Read the model definition and answer for the solid it produces. Units are mm, in the model's axes. Face numbers are marked on the shaded views. Round coordinates to 2 decimals unless told otherwise and drop trailing zeros. Loops run counter-clockwise (first coordinate to the right, second up) from the corner with the lowest first, then second, coordinate; pieces in that order, holes last. Notation, with made-up numbers: (39.5, -8.75) - (54.5, -8.75) arc R11 ccw to (54.5, 10.25) - close; hole circle Ø8 at (-28, 6). An arc over 180 degrees is marked (long way). Answer as CSV lines item,"result".
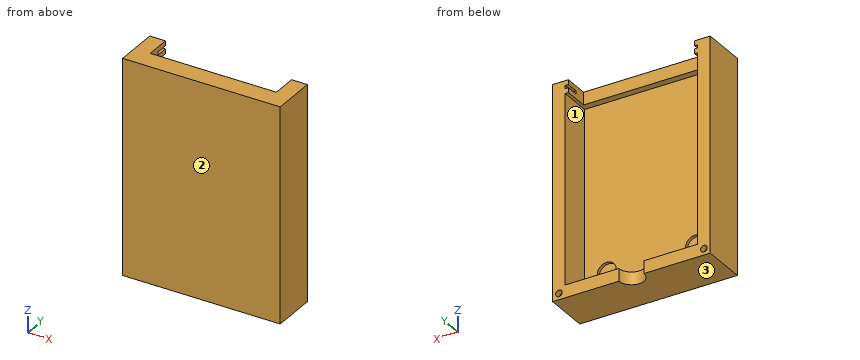
```python
from build123d import *

# Parameters (mm, degrees)
IZIM1_W                     = 25
IZIM1_H                     = 34
Y_KSEKLIK_EKSTR_ZYON1_DEPTH = 7.04
IZIM2_W                     = 21
IZIM2_H                     = 30
KES_EKSTR_ZYON1_DEPTH       = 5.04
IZIM3_W                     = 20
IZIM3_H                     = 3.94
KES_EKSTR_ZYON2_DEPTH       = 36.068669778
FEDER1_START                = -1.1
FEDER1_OUTLINE_W            = 1.1
FEDER1_OUTLINE_H            = 1.1
FEDER1_DEPTH                = 2.2
IZIM7_W                     = 1
IZIM7_H                     = 0.5
KES_EKSTR_ZYON3_DEPTH       = 2
IZIM9_R                     = 2
KES_EKSTR_ZYON4_DEPTH       = 2
IZIM10_R                    = 1.5
KES_EKSTR_ZYON5_DEPTH       = 0.5
IZIM11_R                    = 0.525
KES_EKSTR_ZYON6_DEPTH       = 1.01


# Read off the part's stored shape, not the designer's step: Feder1
with BuildPart() as part:
    # Çizim1 → Yükseklik-Ekstrüzyon1 (new body)
    with BuildSketch(Plane(origin=(0, 7.04, 0), x_dir=(1, 0, 0), z_dir=(0, 1, 0))):
        Rectangle(IZIM1_W, IZIM1_H)
    extrude(amount=-Y_KSEKLIK_EKSTR_ZYON1_DEPTH)

    # Çizim2 → Kes-Ekstrüzyon1 (cut)
    with BuildSketch(Plane(origin=(0, 7.04, 0), x_dir=(-1, 0, 0), z_dir=(0, 1, 0))):
        Rectangle(IZIM2_W, IZIM2_H)
    extrude(amount=-KES_EKSTR_ZYON1_DEPTH, mode=Mode.SUBTRACT)

    # Çizim3 → Kes-Ekstrüzyon2 (cut, through all)
    with BuildSketch(Plane(origin=(0, 0, 15), x_dir=(-1, 0, 0), z_dir=(0, 0, -1))):
        with Locations((0, 5.07)):
            Rectangle(IZIM3_W, IZIM3_H)
    extrude(amount=-KES_EKSTR_ZYON2_DEPTH, mode=Mode.SUBTRACT)

    # Feder1 outline → Feder1 (add)
    with BuildSketch(Plane(origin=(0, 0, 0), x_dir=(0, 0, -1), z_dir=(1, 0, 0)).offset(FEDER1_START)):
        with Locations((14.45, 2.55)):
            Rectangle(FEDER1_OUTLINE_W, FEDER1_OUTLINE_H)
    extrude(amount=FEDER1_DEPTH)

    # Çizim7 → Kes-Ekstrüzyon3 (cut)
    with BuildSketch(Plane(origin=(0, 7.04, 0), x_dir=(1, 0, 0), z_dir=(0, 1, 0))):
        with Locations((-10, -16)):
            Rectangle(IZIM7_W, IZIM7_H)
        with Locations((10, -16)):
            Rectangle(IZIM7_W, IZIM7_H)
    extrude(amount=-KES_EKSTR_ZYON3_DEPTH, mode=Mode.SUBTRACT)

    # Çizim9 → Kes-Ekstrüzyon4 (cut)
    with BuildSketch(Plane(origin=(0, 0, -17), x_dir=(-1, 0, 0), z_dir=(0, 0, -1))):
        with Locations((0, 7.04)):
            Circle(IZIM9_R)
    extrude(amount=-KES_EKSTR_ZYON4_DEPTH, mode=Mode.SUBTRACT)

    # Çizim10 → Kes-Ekstrüzyon5 (cut)
    with BuildSketch(Plane(origin=(0, 2, 0), x_dir=(1, 0, 0), z_dir=(0, 1, 0))):
        with Locations(Location((-7, 11.5, 0), (0, 0, 270))):
            Circle(IZIM10_R)
        with Locations(Location((7, 11.5, 0), (0, 0, 270))):
            Circle(IZIM10_R)
    extrude(amount=-KES_EKSTR_ZYON5_DEPTH, mode=Mode.SUBTRACT)

    # Çizim11 → Kes-Ekstrüzyon6 (cut)
    with BuildSketch(Plane(origin=(0, 7.04, 0), x_dir=(1, 0, 0), z_dir=(0, 1, 0))):
        with Locations(Location((-11.5, 16, 0), (0, 0, 270))):
            Circle(IZIM11_R)
        with Locations(Location((11.5, 16, 0), (0, 0, 270))):
            Circle(IZIM11_R)
    extrude(amount=-KES_EKSTR_ZYON6_DEPTH, mode=Mode.SUBTRACT)


solid = part.part
```
1) A cutting plane is placed at A-A, the plane z = -16. Determine the outline of the cut face in (x, y) (3 decimals).
Entries:
outline,"(-12.5, 0) - (12.5, 0) - (12.5, 7.04) - (12.025, 7.04) - (12.025, 6.03) - (10.975, 6.03) - (10.975, 7.04) - (2, 7.04) arc R2 cw to (-2, 7.04) - (-10.975, 7.04) - (-10.975, 6.03) - (-12.025, 6.03) - (-12.025, 7.04) - (-12.5, 7.04) - close"
2) A cutting plane is placed at D-D, the plane x = -9. Determine the outline of the cut face in (y, z), plus the area to 3 significant figures.
Entries:
outline,"(0, -17) - (7.04, -17) - (7.04, -15) - (2, -15) - (2, 15) - (3.1, 15) - (3.1, 17) - (0, 17) - close"
area,"80.3 mm^2"
3) A cutting plane is placed at B-B, the plane x = 7. Determine the outline of the cut face in (y, z), plus the area to 3 significant figures.
Entries:
outline,"(0, -17) - (7.04, -17) - (7.04, -15) - (2, -15) - (2, -13) - (1.5, -13) - (1.5, -10) - (2, -10) - (2, 15) - (3.1, 15) - (3.1, 17) - (0, 17) - close"
area,"78.8 mm^2"
4) A cutting plane is placed at C-C, the plane z = -11.5. Determine the outline of the cut face in (x, y).
Entries:
outline,"(-12.5, 0) - (12.5, 0) - (12.5, 7.04) - (10.5, 7.04) - (10.5, 2) - (8.5, 2) - (8.5, 1.5) - (5.5, 1.5) - (5.5, 2) - (-5.5, 2) - (-5.5, 1.5) - (-8.5, 1.5) - (-8.5, 2) - (-10.5, 2) - (-10.5, 7.04) - (-12.5, 7.04) - close"
5) Find the intervals of material crossed by line 1 (X direction, y = 1.95, z = -11.5); line 2 (X direction, y = 3.75, z = 8); line 3 (Z direction, x = 1, y = 3), in increasing order.
Entries:
line 1,"x = -12.5 to -8.5, -5.5 to 5.5, 8.5 to 12.5"
line 2,"x = -12.5 to -10.5, 10.5 to 12.5"
line 3,"z = -17 to -13.9, 15 to 17"
6) Each of these flat-tipped pins is pushed along its axis until it touches: P1, Ø0.9, axis at x = -11.5, z = -16, coming from the +Y side; P2, Ø0.6, axis at x = 0, z = -14.5, coming from the +Y side; P3, Ø1.5, axis at x = 3, y = 5, coming from the +Z side. Where does it stop, or does it pass through?
Entries:
P1,"stops at y = 6.03"
P2,"stops at y = 3.1"
P3,"stops at z = -15"
7) The mould has two halves that part along Z. Classify the marked faces 1, 2 and 3: pulls with the +Z half, pulls with the -Z half, needs draft (parallel to the pull), parting line crosses it, or undercut.
Entries:
face 1,"undercut"
face 2,"needs draft"
face 3,"pulls with the -Z half"
